Geometry: final body of the model. Coordinates: model frame, mm. Give positions to 0.01 mm unless a question says otherwise; leave off trailing zeros. Order: outer loops, then holes, each group sorted by start corner. A loop starts at its lowest first (then second) coordinate and runs counter-clockwise, first axis right, second up. Notation, with made-up numbers: M 83,24.25 L 138,24.25 A21 cw 138,44.25 Z; hole C -32.75,-19.75 d4. An arc over 180 degrees is marked long. Use CSV: the item, a comma, the result in double quotes.
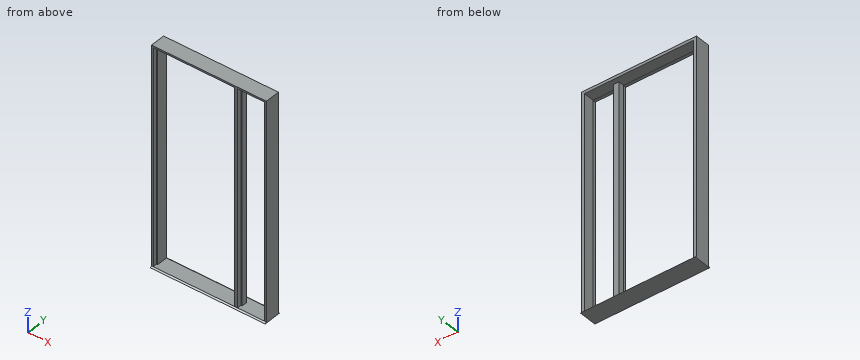
```python
from build123d import *

# Parameters (mm, degrees)
F2_DEPTH      = 2454.275
F4_DEPTH      = 168.276
F6_DEPTH      = 952.5
F6_DEPTH_BACK = 342.9
F8_DEPTH      = 342.9
F8_DEPTH_BACK = 952.5


with BuildPart() as f2:
    # F1 (on Top) → F2 (new body)
    with BuildSketch(Plane.XY):
        Polygon((-952.5, 168.275), (-952.5, 0), (-933.45, 0), (-933.45, 46.0375), (-920.75, 46.0375), (-920.75, 168.275), align=None)
    extrude(amount=F2_DEPTH)


with BuildPart() as f2b:
    # F1 (on Top) → F2, piece 2 (new body)
    with BuildSketch(Plane.XY):
        Polygon((-31.75, 46.0375), (-19.05, 46.0375), (-19.05, 0), (19.05, 0), (19.05, 46.0375), (31.75, 46.0375), (31.75, 111.125), (-31.75, 111.125), align=None)
    extrude(amount=F2_DEPTH)


with BuildPart() as f2c:
    # F1 (on Top) → F2, piece 3 (new body)
    with BuildSketch(Plane.XY):
        Polygon((311.15, 46.0375), (323.85, 46.0375), (323.85, 0), (342.9, 0), (342.9, 168.275), (311.15, 168.275), align=None)
    extrude(amount=F2_DEPTH)


with BuildPart() as f4_tool:
    # F3 (on Front) → F4 (new body, through all)
    with BuildSketch(Plane.XZ):
        Polygon((-31.75, 2454.275), (-952.5, 2454.275), (-492.125, 1993.9), align=None)
        Polygon((342.9, 2454.275), (31.75, 2454.275), (187.325, 2298.7), align=None)
    extrude(amount=-F4_DEPTH)


with BuildPart() as f2_1:
    add(f2.part)

    # F4: cut by f4_tool
    add(f4_tool.part, mode=Mode.SUBTRACT)


    add(f2b.part)  # F6 merges F2b


with BuildPart() as f2c_1:
    add(f2c.part)

    # F4: cut by f4_tool
    add(f4_tool.part, mode=Mode.SUBTRACT)


with BuildPart() as f2_2:
    add(f2_1.part)

    add(f2c_1.part)  # F6 merges F2c
    # F5 (on Right) → F6 (join, two sides)
    with BuildSketch(Plane.YZ) as f6_sk:
        Polygon((168.275, 2422.525), (168.275, 2454.275), (0, 2454.275), (0, 2435.225), (46.0375, 2435.225), (46.0375, 2422.525), align=None)
    extrude(amount=-F6_DEPTH)
    extrude(f6_sk.sketch, amount=F6_DEPTH_BACK)

    # F7 (on Right) → F8 (join, two sides)
    with BuildSketch(Plane.YZ) as f8_sk:
        Polygon((-17.4625, -12.7), (84.1375, -12.7), (185.7375, -12.7), (169.8625, 0), (84.1375, 0), (-1.5875, 0), align=None)
    extrude(amount=F8_DEPTH)
    extrude(f8_sk.sketch, amount=-F8_DEPTH_BACK)


solid = f2_2.part
```
1. Pin query (flat end, axial travel): pin 1 Ø6 at (x, z) = (-32, 534.5) entering from +Y (3 decimals). Return the tip coordinate at first contact, or that it passes through.
Answer:
pin 1,"y = 111.125"
2. Line query: line 1 (X direction, y = 14, z = 1966); line 2 (X direction, y = 64.5, z = 2223); line 3 (X direction, y = 146, z = 1663.5). Output: solid intervals per line, ascending.
Answer:
line 1,"-952.5 to -933.45, -19.05 to 19.05, 323.85 to 342.9"
line 2,"-952.5 to -920.75, -31.75 to 31.75, 311.15 to 342.9"
line 3,"-952.5 to -920.75, 311.15 to 342.9"
3. Section A-A, the plane x = -119.5. Return the cut outline in (y, z) (1 decimal).
Answer:
outline,"M -17.5,-12.7 L 185.7,-12.7 L 169.9,0 L -1.6,0 Z; M 0,2435.2 L 46,2435.2 L 46,2422.5 L 168.3,2422.5 L 168.3,2454.3 L 0,2454.3 Z"
4. Section B-B, the plane z = 2250. Give the number of separate pieces and of enclosed holes in the cut face, plus the area to 3 significant figures.
Answer:
separate pieces,"3"
enclosed holes,"0"
area,"15,400 mm2"
5. Section C-C, the plane y = 88.5. Return the cut outline in (x, z) (3 decimals).
Answer:
outline,"M -952.5,-12.7 L 342.9,-12.7 L 342.9,2454.275 L -952.5,2454.275 Z; hole M -920.75,0 L -31.75,0 L -31.75,2422.525 L -920.75,2422.525 Z; hole M 31.75,0 L 311.15,0 L 311.15,2422.525 L 31.75,2422.525 Z"
